Geometry: final body of the model. Coordinates: model frame, mm. A direction names the side the tool comes from. Give positions to 0.01 mm unless a question says otherwise; leave off trailing zeros. Loops run counter-clockwise (first coordinate to the right, second up) from the corner with the lowest first, then second, coordinate; pieces in that order, holes last.
from build123d import *

# Parameters (mm, degrees)
SKETCH1_W              = 200
SKETCH1_H              = 22
BOSS_EXTRUDE1_DEPTH    = 1
SKETCH2_W              = 200
SKETCH2_H              = 6.5
BOSS_EXTRUDE2_DEPTH    = 6
SKETCH5_R              = 2.3
SLOT_1_DEPTH           = 101.781942827
SLOT_2_COPY_1_SKETCH_R = 2.3
SLOT_2_COPY_1_DEPTH    = 101.781942827
DEBURS_SIZE            = 0.2


with BuildPart() as part:
    # Sketch1 → Boss-Extrude1 (new body)
    with BuildSketch(Plane.XY):
        Rectangle(SKETCH1_W, SKETCH1_H)
    extrude(amount=-BOSS_EXTRUDE1_DEPTH)

    # Sketch2 → Boss-Extrude2 (add)
    with BuildSketch(Plane.XY):
        with Locations((0, 7.75)):
            Rectangle(SKETCH2_W, SKETCH2_H)
        with Locations((0, -7.75)):
            Rectangle(SKETCH2_W, SKETCH2_H)
    extrude(amount=BOSS_EXTRUDE2_DEPTH)

    # Sketch5 → Slot 1 (cut, symmetric)
    with BuildSketch(Plane(origin=(0, 0, 0), x_dir=(0, 0, -1), z_dir=(1, 0, 0))):
        with Locations((-3.25, 4.5)):
            Circle(SKETCH5_R)
    slot_1 = extrude(amount=SLOT_1_DEPTH, both=True, mode=Mode.SUBTRACT)

    # Slot 1x2: Slot 1 across plane
    add(slot_1.mirror(Plane(origin=(0, 7.75, 0), x_dir=(0, 0, 1), z_dir=(0, -1, 0))), mode=Mode.SUBTRACT)

    # Slot 2: Slot 1 across plane
    add(slot_1.mirror(Plane.ZX), mode=Mode.SUBTRACT)

    # Slot 2 copy 1 sketch → Slot 2 copy 1 (cut, symmetric)
    with BuildSketch(Plane(origin=(0, -15.5, 0), x_dir=(0, 0, -1), z_dir=(1, 0, 0))):
        with Locations((-3.25, 4.5)):
            Circle(SLOT_2_COPY_1_SKETCH_R)
    extrude(amount=SLOT_2_COPY_1_DEPTH, both=True, mode=Mode.SUBTRACT)

    # Deburs
    deburs_edges = [part.edges().sort_by_distance(p)[0] for p in [
        (0, 11, -1),
        (0, -11, -1),
    ]]
    chamfer(deburs_edges, length=DEBURS_SIZE)


solid = part.part
Item 1: Set-up query: faces 1 (the face through (1.4, -6.8, 3.2)), 2 (the face through (1.4, -8.7, 3.2)). Return all of +Z, -Z, +X, -X, +Y, -Y with unobstructed straight access to the full face (end or side cutting, diameter ignored); none if empty.
Values follow:
face 1: +X, -X
face 2: +X, -X, -Y
Item 2: Ray query, probe 1 along Y at (x, z) = (-67.5, 5.75); probe 2 along Y at (x, z) = (-53, 3); probe 3 along Z at (x, y) = (-40, -1.5). Return the intervals inside material, ascending.
Values follow:
probe 1: y = -11 to -4.5, 4.5 to 11
probe 2: y = -8.71 to -6.79, 6.79 to 8.71
probe 3: z = -1 to 0
Item 3: Pin query (flat end, axial travel): pin 1 (10 mm diameter, centred on x = 35, y = 1.5, fed in from +Z); pin 2 (2 mm diameter, centred on x = 54.5, z = 3.5, fed in from -Y). Return the tip coordinate at first contact, or that it passes through.
Values follow:
pin 1: stops at z = 6
pin 2: stops at y = -9.07
Item 4: Draft query along Z for faces 3 (the face through (-1, 0, 0)), 4 (the face through (-100, -0.2, -0.7)), 5 (the face through (1.4, 6.8, 3.2)). Return one class per face: +Z half, -Z half, draft (parallel to the pull), parting line (faces both ways), or undercut.
Values follow:
face 3: +Z half
face 4: draft
face 5: undercut
Item 5: Section query C-C on y = 2. Return loops of the section in (x, z), plus the area to 3 significant figures.
Values follow:
outline: (-100, -1) - (100, -1) - (100, 0) - (-100, 0) - close
area: 200 mm2
Item 6: Section query A-A on z = 3. Return loops of the section in (x, y).
Values follow:
outline: (-100, -8.71) - (100, -8.71) - (100, -6.79) - (-100, -6.79) - close; (-100, 6.79) - (100, 6.79) - (100, 8.71) - (-100, 8.71) - close
Item 7: Section query B-B on x = -48. Return loops of the section in (y, z), plus the area to 3 significant figures.
Values follow:
outline: (-11, -0.8) - (-10.8, -1) - (10.8, -1) - (11, -0.8) - (11, 0.95) arc R2.3 cw to (11, 5.55) - (11, 6) - (4.5, 6) - (4.5, 5.55) arc R2.3 cw to (4.5, 0.95) - (4.5, 0) - (-4.5, 0) - (-4.5, 0.95) arc R2.3 cw to (-4.5, 5.55) - (-4.5, 6) - (-11, 6) - (-11, 5.55) arc R2.3 cw to (-11, 0.95) - close
area: 66.7 mm2
